```python
from build123d import *

# Parameters (mm, degrees)
SKETCH1_W                    = 50
SKETCH1_H                    = 16
BOSS_EXTRUDE1_DEPTH          = 5
SKETCH2_W                    = 7
SKETCH2_H                    = 14
F_5_0_5_DIAMETER_HOLE1_D     = 5
F_5_0_5_DIAMETER_HOLE1_DEPTH = 12
CHAMFER1_SIZE                = 2.5
CHAMFER2_SIZE                = 2
SKETCH5_R                    = 17.5
BOSS_EXTRUDE2_DEPTH          = 7


with BuildPart() as part:
    # Sketch1 → Boss-Extrude1 (new body)
    with BuildSketch(Plane(origin=(5, 0, 0), x_dir=(0, 0, -1), z_dir=(1, 0, 0))):
        Rectangle(SKETCH1_W, SKETCH1_H)
    extrude(amount=-BOSS_EXTRUDE1_DEPTH)

    # Sketch2 → Revolve1 (revolve)
    with BuildSketch(Plane(origin=(0, 0, 0), x_dir=(-1, 0, 0), z_dir=(0, 0, -1)), mode=Mode.PRIVATE) as revolve1_sk:
        with Locations((3.5, 7)):
            Rectangle(SKETCH2_W, SKETCH2_H)
    revolve(revolve1_sk.sketch.rotate(Axis((0, 0, 0), (-1, 0, 0)), 270), axis=Axis((0, 0, 0), (-1, 0, 0)))

    # Ø5.0 (5) Diameter Hole1
    with Locations(Plane(origin=(5, 0, 0), x_dir=(0, 0, -1), z_dir=(1, 0, 0))):
        with Locations((-20, 0), (20, 0)):
            Hole(F_5_0_5_DIAMETER_HOLE1_D / 2, depth=F_5_0_5_DIAMETER_HOLE1_DEPTH)

    # Chamfer1
    chamfer1_edges = [part.edges().sort_by_distance(p)[0] for p in [
        (2.5, 8, 25),
        (2.5, 8, -25),
        (2.5, -8, -25),
    ]]
    chamfer(chamfer1_edges, length=CHAMFER1_SIZE)

    # Chamfer2
    chamfer2_edges = [part.edges().sort_by_distance(p)[0] for p in [
        (2.5, -8, 25),
    ]]
    chamfer(chamfer2_edges, length=CHAMFER2_SIZE)

    # Sketch5 → Boss-Extrude2 (add)
    with BuildSketch(Plane.ZY.offset(7)):
        Circle(SKETCH5_R)
    extrude(amount=-BOSS_EXTRUDE2_DEPTH)


solid = part.part
```
Read the model definition and answer for the solid it produces. Units are mm, in the model's axes. A direction names the side the tool comes from. Coordinates: 2 decimals unless noted, no trailing zeros. Loops run counter-clockwise (first coordinate to the right, second up) from the corner with the lowest first, then second, coordinate; pieces in that order, holes last.
(1) Consider line 1 along Y through (x, z) = (1.2, 20); line 2 along X through (y, z) = (-16, 5); line 3 along Z through (x, y) = (-2.75, 6). Determine where each line is inside the solid, lowest interval first.
Solution:
line 1: y = -8 to -2.5, 2.5 to 8
line 2: x = -7 to 0
line 3: z = -16.44 to 16.44
(2) The part is cut by section A-A (y = 0.5). Determine the outline of the cut face in (x, z).
Solution:
outline: (-7, -17.49) - (0, -17.49) - (0, -17.55) - (5, -17.55) - (5, 17.55) - (0, 17.55) - (0, 17.49) - (-7, 17.49) - close; (0, -25) - (5, -25) - (5, -22.45) - (0, -22.45) - close; (0, 22.45) - (5, 22.45) - (5, 25) - (0, 25) - close
(3) The part is cut by section B-B (x = 3.5). Determine the outline of the cut face in (y, z).
Solution:
outline: (-8, -22.5) - (-5.5, -25) - (5.5, -25) - (8, -22.5) - (8, 22.5) - (5.5, 25) - (-6, 25) - (-8, 23) - close; hole circle Ø5 at (0, -20); hole circle Ø5 at (0, 20)
(4) The part is cut by section D-D (z = -13.5). Determine the outline of the cut face in (x, y), and give its area (3 significant figures).
Solution:
outline: (-7, -11.14) - (0, -11.14) - (0, -8) - (5, -8) - (5, 8) - (0, 8) - (0, 11.14) - (-7, 11.14) - close
area: 236 mm2
(5) The part is cut by section C-C (z = 20). Determine the outline of the cut face in (x, y), and give its area (3 significant figures).
Solution:
outline: (0, -8) - (5, -8) - (5, -2.5) - (0, -2.5) - close; (0, 2.5) - (5, 2.5) - (5, 8) - (0, 8) - close
area: 55.0 mm2
(6) The mould has two halves that part along Y. Classify faces 1 (the face through (0, 2, -22)), 2 (the face through (2.5, 0.1, 17.5)), 3 (the face through (-3.549, -10.648, -13.887)), 4 (the face through (3, -8, 1)): released by +Y, released by -Y, zero draft, split by the parting line, or undercut.
Solution:
face 1: zero draft
face 2: undercut
face 3: split by the parting line
face 4: released by -Y
(7) Flat-ended cylindrical pins translate along their axes: pin 1 Ø5 at (x, z) = (-1.5, 10.5) entering from -Y; pin 2 Ø3 at (y, z) = (-3, -20.5) entering from -X; pin 3 Ø3 at (x, y) = (-2, 9.5) entering from +Z; pin 4 Ø6.5 at (y, z) = (0, -20) entering from -X. Find the tip coordinate at first contact, or state that the pin passes through.
Solution:
pin 1: stops at y = -15.56
pin 2: stops at x = 0
pin 3: stops at z = 15.56
pin 4: stops at x = -7
(8) A tool of negligible diameter and unlimited length cuts with its end or side. For faces 5 (the face through (3, 0, 25)), 6 (the face through (0, -12, 0)), 7 (the face through (0, 12, 0)), from which of +Z, -Z, +X, -X, +Y, -Y can it reach the whole face along a straight path? Write none if from no direction.
Solution:
face 5: +Z, +X, -X, +Y, -Y
face 6: +Z, -Z, +X, -Y
face 7: +Z, -Z, +X, +Y
